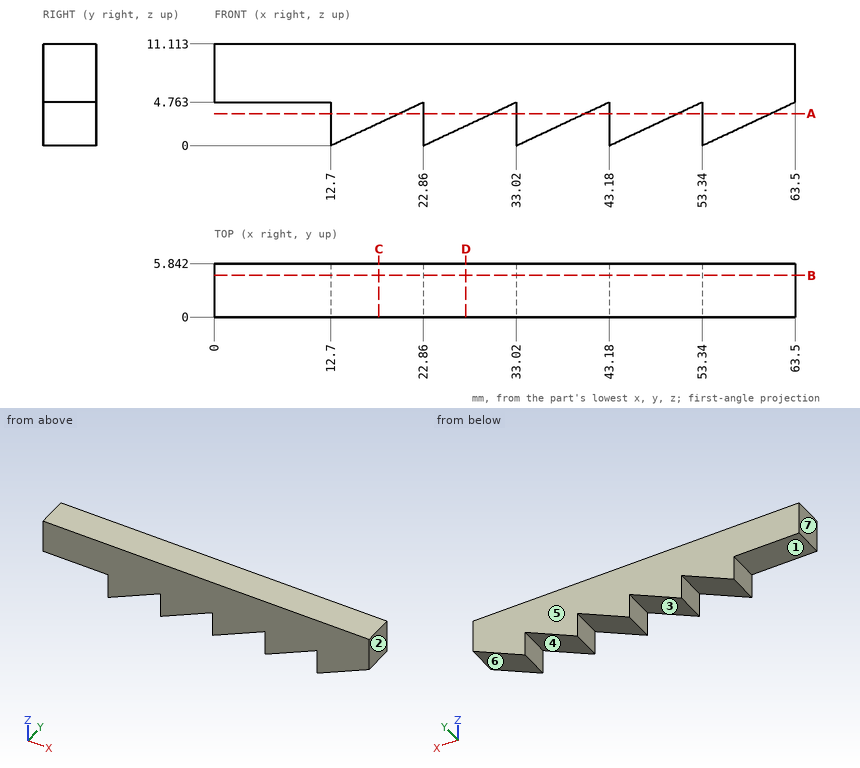
Input: dimensioned drawing with shaded views. Units: mm. Origin: part minimum x, y, z. A direction names the side the tool comes from. Give positions to 0.01 mm unless a question says otherwise; leave off trailing zeros. Write each loop counter-clockwise with the first axis right and the second up, starting at its lowest first coordinate (ties: lowest second). Pieces come first, ordered by that corner, then holes.
Q1. Section A-A, the plane z = 3.5. Output: boundary loops of the cut face in (x, y).
Q2. Material intervals for probe 1 along X at (y, z) = (3.6, 4.5) (1 decimal); probe 2 along X at (y, z) = (3, 3) (1 decimal); probe 3 along Z at (x, y) = (5.5, 1), sorted ascending.
Q3. Section B-B, the plane y = 4.55. Output: boundary loops of the cut face in (x, z), plus the area to 3 significant figures.
Q4. Section C-C, the plane x = 18. Output: boundary loops of the cut face in (y, z) (1 decimal), plus the area to 3 significant figures.
Q5. Set-up query: the marked faces 1, 2 and 3. Return all of +Z, -Z, +X, -X, +Y, -Y with unobstructed straight access to the full face (end or side cutting, diameter ignored); none if empty.
Q6. Section D-D, the plane x = 27.5. Output: boundary loops of the cut face in (y, z) (1 decimal).
Q7. Pull-direction query (X, two-part tool) for the marked faces 4, 5, 6 and 7; classes: pulls with the +X half, pulls with the -X half, needs draft (parallel to the pull), parting line crosses it, or undercut.
Q8. First-contact query: P1, Ø1.4, axis at y = 3.5, z = 2, coming from the -X side; P2, Ø1.8, axis at x = 8, y = 4.5, coming from the -Z side. Flat tips, straight axial feed; report the tip coordinate or a pass-through.
Filled in:
1. outline: (12.7, 0) - (20.17, 0) - (20.17, 5.84) - (12.7, 5.84) - close; (22.86, 0) - (30.33, 0) - (30.33, 5.84) - (22.86, 5.84) - close; (33.02, 0) - (40.49, 0) - (40.49, 5.84) - (33.02, 5.84) - close; (43.18, 0) - (50.65, 0) - (50.65, 5.84) - (43.18, 5.84) - close; (53.34, 0) - (60.81, 0) - (60.81, 5.84) - (53.34, 5.84) - close
2. probe 1: x = 12.7 to 22.3, 22.9 to 32.5, 33 to 42.6, 43.2 to 52.8, 53.3 to 62.9
2. probe 2: x = 12.7 to 19.1, 22.9 to 29.3, 33 to 39.4, 43.2 to 49.6, 53.3 to 59.7
2. probe 3: z = 4.76 to 11.11
3. outline: (0, 4.76) - (12.7, 4.76) - (12.7, 0) - (22.86, 4.76) - (22.86, 0) - (33.02, 4.76) - (33.02, 0) - (43.18, 4.76) - (43.18, 0) - (53.34, 4.76) - (53.34, 0) - (63.5, 4.76) - (63.5, 11.11) - (0, 11.11) - close
3. area: 524 mm2
4. outline: (0, 2.5) - (5.8, 2.5) - (5.8, 11.1) - (0, 11.1) - close
4. area: 50.4 mm2
5. face 1: -Z, -X, +Y, -Y
5. face 2: +Z, -Z, +X, +Y, -Y
5. face 3: -Z, +Y, -Y
6. outline: (0, 2.2) - (5.8, 2.2) - (5.8, 11.1) - (0, 11.1) - close
7. face 4: undercut
7. face 5: needs draft
7. face 6: pulls with the +X half
7. face 7: pulls with the -X half
8. P1: stops at x = 12.7
8. P2: stops at z = 4.76
